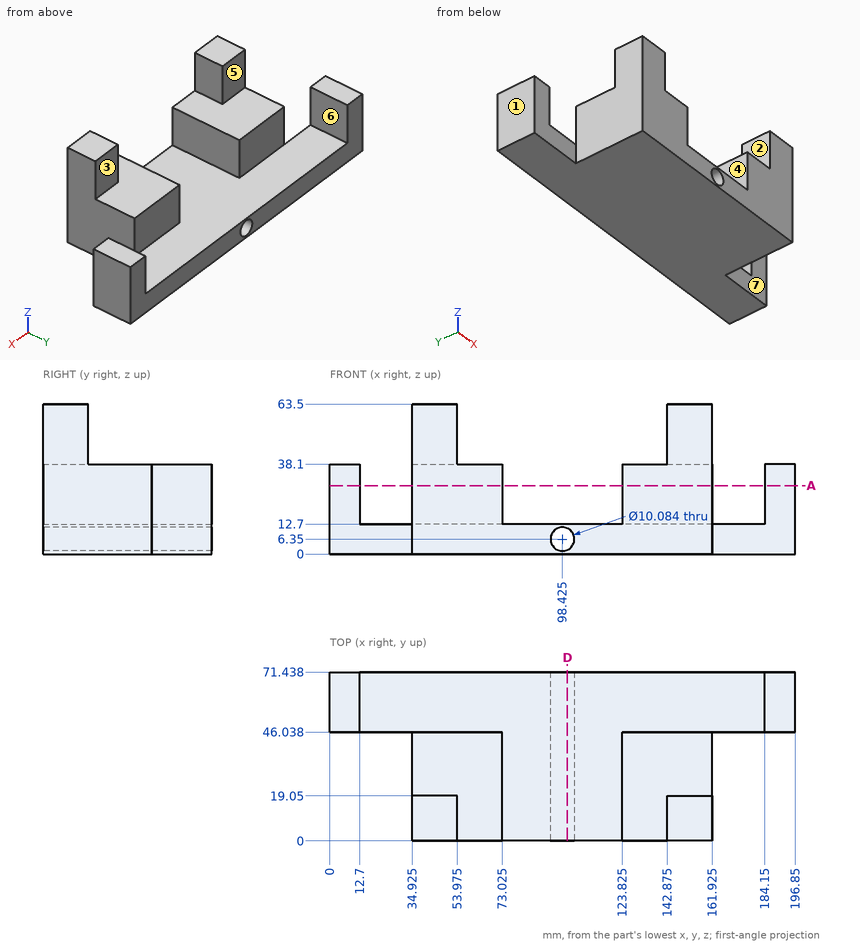
The drawing under review shows one solid part. Ordinate dimensions are in mm from its lowest x, y, z. A direction names the side the tool comes from. Round coordinates to 2 decimals unless told otherwise and drop trailing zeros. Loops run counter-clockwise (first coordinate to the right, second up) from the corner with the lowest first, then second, coordinate; pieces in that order, holes last. Notation, with made-up numbers: (-19.75, 82.5) - (-7.75, 82.5) arc R25 ccw to (-7.75, 112.5) - close; hole circle Ø1 at (51, -38). An arc over 180 degrees is marked (long way). Use a Markdown table: item, result. Add a question column.
Q1. The part is to be moulded in two halves that separate along X. For the marked faces 1, 2, 3 and 4, say which applies: pulls with the +X half, pulls with the -X half, needs draft (parallel to the pull), parting line crosses it, or undercut.
Q2. Add section D-D (x = 100.5). State the section outline as (y, z) points (1 decimal).
Q3. Machinability: for the marked faces 5, 6 and 7, which of the approach directions +Z, -Z, +X, -X, +Y, -Y give a long, thin tool a straight path to every point of the face, cutting with its end or side? Answer none if there is none.
Q4. Add section A-A (z = 29). State how many separate pieces and enclosed holes the cut face has, plus the area to 3 significant figures.
Q5. For probe 1 along X at (y, z) = (59.5, 17); probe 2 along X at (y, z) = (19, 30.5) (1 decimal); probe 3 along Z at (x, y) = (142.5, 60.5), list the stretches that pass through material, from the lowest coordinate up.
Q6. Insertion check: pin 1 Ø15 at (y, z) = (12.5, 52.5) entering from -X (1 decimal); pin 2 Ø7.5 at (x, z) = (63, 29) entering from +Y; pin 3 Ø1 at (x, y) = (64, 29) entering from +Z; pin 4 Ø6 at (y, z) = (25, 48.5) entering from -X. Each pin has a flat end and moves straight along its axis. Give the tip position at first contact, or say it passes through.
Worked answers:
| question | item | result |
|---|---|---|
| 1 | face 1 | pulls with the -X half |
| 1 | face 2 | undercut |
| 1 | face 3 | needs draft |
| 1 | face 4 | undercut |
| 2 | outline | (0, 0) - (71.4, 0) - (71.4, 1.8) - (0, 1.8) - close; (0, 10.9) - (71.4, 10.9) - (71.4, 12.7) - (0, 12.7) - close |
| 3 | face 5 | +Z, +X, -X, +Y |
| 3 | face 6 | +Z, +Y, -Y |
| 3 | face 7 | +Z, -Z, +X, -Y |
| 4 | separate pieces | 4 |
| 4 | enclosed holes | 0 |
| 4 | area | 4,150 mm² |
| 5 | probe 1 | 0 to 12.7, 184.15 to 196.85 |
| 5 | probe 2 | 34.9 to 73, 123.8 to 161.9 |
| 5 | probe 3 | 0 to 12.7 |
| 6 | pin 1 | x = 34.9 |
| 6 | pin 2 | y = 46.04 |
| 6 | pin 3 | z = 38.1 |
| 6 | pin 4 | through |
